Verification items for the finished model (mm, model axes). A direction names the side the tool comes from. Coordinates: 2 decimals unless noted, no trailing zeros. Order: outer loops, then holes, each group sorted by start corner. A loop starts at its lowest first (then second) coordinate and runs counter-clockwise, first axis right, second up.
Q1. Set-up check for faces 1 (the flat face through (9.86, 110.58, -25.29)), 2 (the cylindrical face through (-18.496, 104.518, -27.595)), 3 (the cylindrical face through (8.82, 107.28, -41.43)), 4 (the flat face through (-9.86, 112.244, -16.363)): record each of +Z, -Z, +X, -X, +Y, -Y from which the full face is reachable in a straight line by a thin tool's end or side.
Q2. Draft check along Z on faces 5 (the flat face through (0, 110, 0)), 6 (the cylindrical face through (-13.4, 114.52, -10.51)), 7 (the flat face through (6.286, 99.587, -54.424)). Enter one of: pulls with the +Z half, pulls with the -Z half, needs draft (parallel to the pull), parting line crosses it, or undercut.
Q3. Thickness scan on line 1 (X direction, y = 113.75, z = -8); line 2 (X direction, y = 107.5, z = -35.5) (3 decimals); line 3 (X direction, y = 104, z = -42.5). Record the ranges inside material, lowest first.
Q4. Depth check by flat-ended pin: P1, Ø5, axis at x = 2, y = 95.5, coming from the -Z side; P2, Ø3, axis at x = 5, z = -24, coming from the +Y side; P3, Ø1.5, axis at x = 11, y = 105, coming from the -Z side. Enter the tip coordinate at first touch or a pass-through.
Q5. Cross-section at A-A, the plane x = 13. Record the boundary of the cut face in (y, z) (3 decimals), and give its area (3 significant figures).
from build123d import *
from build123d.topology import SkipClean

# Parameters (mm, degrees)
CUT_EXTRUDE1_REACH      = 261.709
CUT_EXTRUDE1_END_RADIUS = 112
CIRPATTERN1_COUNT       = 34
SKETCH5_OUTSIDE_W       = 297.544
SKETCH5_OUTSIDE_H       = 297.544
CUT_EXTRUDE2_DEPTH      = 168.481342244


with BuildPart() as part:
    # Sketch1 → Revolve1 (revolve)
    with BuildSketch(Plane.XY, mode=Mode.PRIVATE) as revolve1_sk:
        Polygon((-20, 115), (20, 115), (20, 108.1), (16.95, 108.1), (13.9, 105.05), (-16.95, 105.05), (-16.95, 108.1), (-20, 108.1), align=None)
    revolve(revolve1_sk.sketch.rotate(Axis((22, 0, 0), (-1, 0, 0)), 90), axis=Axis((22, 0, 0), (-1, 0, 0)))

    # Cut-Extrude1: up to this cylinder (the profile starts outside it)
    cut_extrude1_end = Plane(origin=(0, 0, 0), z_dir=(-1, 0, 0)) * Cylinder(CUT_EXTRUDE1_END_RADIUS, 748.418, mode=Mode.PRIVATE)
    # Sketch3 → Cut-Extrude1 (cut, up to the surface)
    with BuildSketch(Plane.XY.offset(117), mode=Mode.PRIVATE) as cut_extrude1_sk1:
        Polygon((-20, 7.5), (-3.333333333, 0), (-20, -7.5), (-20, -10.5), (0, -1.5), (20, -10.5), (20, -7.5), (3.333333333, 0), (20, 7.5), (20, 10.5), (0, 1.5), (-20, 10.5), align=None)
    cut_extrude1_tool1 = extrude(cut_extrude1_sk1.sketch, amount=-CUT_EXTRUDE1_REACH, mode=Mode.PRIVATE) - cut_extrude1_end
    cut_extrude1 = cut_extrude1_tool1.solids().sort_by_distance((0, 0, 117))[0]
    add(cut_extrude1, mode=Mode.SUBTRACT)

    # CirPattern1: Cut-Extrude1 ×34 about axis
    with SkipClean():  # the faces are left unmerged after this step: merging them gives an invalid solid
        cirpattern1_axis = Axis((0, 0, 0), (1, 0, 0))
        for i in range(1, CIRPATTERN1_COUNT):
            add(cut_extrude1.rotate(cirpattern1_axis, i * 360 / CIRPATTERN1_COUNT), mode=Mode.SUBTRACT)

    # Sketch4 → Cut-Revolve1 (revolve, cut)
    with SkipClean():  # the faces are left unmerged after this step: merging them gives an invalid solid
        with BuildSketch(Plane.XY, mode=Mode.PRIVATE) as cut_revolve1_sk:
            Polygon((-1.5, 115), (1.5, 115), (0, 112), align=None)
        revolve(cut_revolve1_sk.sketch.rotate(Axis((22, 0, 0), (-1, 0, 0)), 270), axis=Axis((22, 0, 0), (-1, 0, 0)), mode=Mode.SUBTRACT)

    # Sketch5 outside → Cut-Extrude2 (cut, through all)
    with BuildSketch(Plane.ZY.offset(20)):
        Rectangle(SKETCH5_OUTSIDE_W, SKETCH5_OUTSIDE_H)
        with BuildLine():
            Line((0, 0), (0, 124.880273578))
            ThreePointArc((0, 124.880273578), (-34.133726301, 125.732826073), (-66.737856602, 115.593358423))
            Line((-66.737856602, 115.593358423), (0, 0))
        make_face(mode=Mode.SUBTRACT)
    extrude(amount=-CUT_EXTRUDE2_DEPTH, mode=Mode.SUBTRACT)


solid = part.part
Check values:
1. face 1: none
1. face 2: +Z, -X, -Y
1. face 3: -Z, +X, -X, +Y
1. face 4: +Y
2. face 5: pulls with the +Z half
2. face 6: pulls with the -Z half
2. face 7: undercut
3. line 1: x = -20 to -8.95, -2.29 to -1.02, 1.02 to 2.29, 8.95 to 20
3. line 2: x = -20 to -13.836, -7.169 to -0.605, 0.605 to 7.169, 13.836 to 20
3. line 3: x = -15.14 to -0.17, 0.17 to 15.14
4. P1: stops at z = -56.58
4. P2: stops at y = 112.78
4. P3: stops at z = -48.55
5. outline: (90.976, -52.525) - (96.995, -56) arc R112 ccw to (98.244, -53.779) - (100.931, -55.117) arc R115 ccw to (104.809, -47.329) - (102.122, -45.991) arc R112 ccw to (103.318, -43.236) - (106.009, -44.576) arc R115 ccw to (108.372, -38.476) - (105.481, -37.654) arc R112 ccw to (106.453, -34.811) - (109.34, -35.633) arc R115 ccw to (111.721, -27.265) - (108.834, -26.443) arc R112 ccw to (109.504, -23.515) - (112.395, -24.337) arc R115 ccw to (113.597, -17.908) - (110.604, -17.63) arc R112 ccw to (111.037, -14.658) - (114.026, -14.935) arc R115 ccw to (114.829, -6.272) - (111.839, -5.995) arc R112 ccw to (111.96, -2.993) - (114.953, -3.271) arc R115 ccw to (115, 0) - (105.05, 0) arc R105.05 cw to start
5. area: 520 mm2
